from build123d import *

# Parameters (mm, degrees)
F0_W     = 482.6
F0_H     = 43.7
F1_DEPTH = 3
F2_W     = 3.5
F2_H     = 6.8
F3_W     = 3.5
F3_H     = 6.8
F4_DEPTH = 3
F6_DEPTH = 3


with BuildPart() as f1:
    # F0 (on Front) → F1 (new body)
    with BuildSketch(Plane.XZ):
        Rectangle(F0_W, F0_H)
    extrude(amount=-F1_DEPTH)

    # F2 (on face) + F3 (on face) → F4 (cut)
    with BuildSketch(Plane.XZ):
        with Locations((-232.5, 0)):
            Rectangle(F2_W, F2_H)
        with BuildLine():
            Line((-230.75, 3.4), (-230.75, -3.4))
            ThreePointArc((-230.75, -3.4), (-227.35, 0), (-230.75, 3.4))
        make_face()
        with BuildLine():
            ThreePointArc((-234.25, 3.4), (-237.65, 0), (-234.25, -3.4))
            Line((-234.25, -3.4), (-234.25, 3.4))
        make_face()
    with BuildSketch(Plane.XZ):
        with Locations((232.5, 0)):
            Rectangle(F3_W, F3_H)
        with BuildLine():
            Line((234.25, 3.4), (234.25, -3.4))
            ThreePointArc((234.25, -3.4), (237.65, 0), (234.25, 3.4))
        make_face()
        with BuildLine():
            ThreePointArc((230.75, 3.4), (227.35, 0), (230.75, -3.4))
            Line((230.75, -3.4), (230.75, 3.4))
        make_face()
    extrude(amount=-F4_DEPTH, mode=Mode.SUBTRACT)

    # F5 (on face) → F6 (cut)
    with BuildSketch(Plane.XZ):
        with BuildLine():
            ThreePointArc((106.6389867841, -1.5694810542), (107.9654749762, -1.2364507967), (108.55, 0))
            ThreePointArc((108.55, 0), (107.9654749762, 1.2364507967), (106.6389867841, 1.5694810542))
            ThreePointArc((106.6389867841, 1.5694810542), (106.7222120696, 0.7867011367), (106.75, 0))
            ThreePointArc((106.75, 0), (106.7222120696, -0.7867011367), (106.6389867841, -1.5694810542))
        make_face()
        with BuildLine():
            ThreePointArc((106.75, 0), (106.7222120696, 0.7867011367), (106.6389867841, 1.5694810542))
            ThreePointArc((106.6389867841, 1.5694810542), (105.35, 0), (106.6389867841, -1.5694810542))
            ThreePointArc((106.6389867841, -1.5694810542), (106.7222120696, -0.7867011367), (106.75, 0))
        make_face()
        with BuildLine():
            ThreePointArc((106.6389867841, -1.5694810542), (105.35, 0), (106.6389867841, 1.5694810542))
            ThreePointArc((106.6389867841, 1.5694810542), (84.45, 0), (106.6389867841, -1.5694810542))
        make_face()
    extrude(amount=-F6_DEPTH, mode=Mode.SUBTRACT)


solid = f1.part
Read the model definition and answer for the solid it produces. Units are mm, in the model's axes. Round coordinates to 2 decimals unless told otherwise and drop trailing zeros. Order: outer loops, then holes, each group sorted by start corner. A loop starts at its lowest first (then second) coordinate and runs counter-clockwise, first axis right, second up.
1) The part is cut by section A-A on x = 95.6. Write down the section's boundary in (y, z), plus the area to 3 significant figures.
2) The part is cut by section B-B on y = 1.4. Write down the section's boundary in (x, z).
3) The mould has two halves that part along Z. Classify faces 1 (the face through (-3, 3, 0)), 2 (the face through (84.46, 1.48, 0.47)): released by +Z, released by -Z, zero draft, split by the parting line, or undercut.
4) Straight lines are drawn through the part: L1, parallel to Z at x = 95.6, y = 1.6; L2, parallel to X at y = 1.85, z = 2; L3, parallel to X at y = 1.5, z = -2.5. For each, find the intervals that lie inside material, in ascending order.
Resolved:
1. outline: (0, -21.85) - (3, -21.85) - (3, -11.15) - (0, -11.15) - close; (0, 11.15) - (3, 11.15) - (3, 21.85) - (0, 21.85) - close
1. area: 64.2 mm2
2. outline: (-241.3, -21.85) - (241.3, -21.85) - (241.3, 21.85) - (-241.3, 21.85) - close; hole (-234.25, -3.4) - (-230.75, -3.4) arc R3.4 ccw to (-230.75, 3.4) - (-234.25, 3.4) arc R3.4 ccw to start; hole (106.64, -1.57) arc R1.6 ccw (long way) to (106.64, 1.57) arc R11.15 ccw (long way) to start; hole (230.75, -3.4) - (234.25, -3.4) arc R3.4 ccw to (234.25, 3.4) - (230.75, 3.4) arc R3.4 ccw to start
3. face 1: zero draft
3. face 2: undercut
4. L1: z = -21.85 to -11.15, 11.15 to 21.85
4. L2: x = -241.3 to -237, -228 to 84.63, 106.57 to 228, 237 to 241.3
4. L3: x = -241.3 to -236.55, -228.45 to 84.73, 106.47 to 228.45, 236.55 to 241.3
